from build123d import *

# Parameters (mm, degrees)
SKETCH_1_R          = 9
EXTRUDE_1_DEPTH     = 20
EXTRUDE_START       = 10
SKETCH_2_R          = 9
EXTRUDE_2_DEPTH     = 10
SKETCH_4_R          = 5.45
SKETCH_4_R_2        = 2.8
CUT_EXTRUDE_1_DEPTH = 7
SKETCH_5_R          = 2.9
EXTRUDE_3_DEPTH     = 10
CHAMFER_1_SIZE      = 0.6
CHAMFER_2_SIZE      = 0.4
FILLET_3_R          = 0.4


with BuildPart() as part:
    # 草图1 → 凸台-拉伸1 (new body)
    with BuildSketch(Plane(origin=(0, 0, 0), x_dir=(0, 0, -1), z_dir=(1, 0, 0))):
        Circle(SKETCH_1_R)
        with BuildLine():
            Line((-2.2, 4.4), (2.2, 4.4))
            Line((2.2, 4.4), (2.2, 6.8556546))
            ThreePointArc((2.2, 6.8556546), (0, -7.2), (-2.2, 6.8556546))
            Line((-2.2, 6.8556546), (-2.2, 4.4))
        make_face(mode=Mode.SUBTRACT)
    extrude(amount=-EXTRUDE_1_DEPTH)

    # 草图2 → 凸台-拉伸2 (add)
    with BuildSketch(Plane(origin=(0, 0, 0), x_dir=(0, 0, -1), z_dir=(1, 0, 0)).offset(EXTRUDE_START)):
        Circle(SKETCH_2_R)
    extrude(amount=-EXTRUDE_2_DEPTH)

    # 草图4 → 切除-拉伸1 (cut)
    with BuildSketch(Plane(origin=(10, 0, 0), x_dir=(0, 0, -1), z_dir=(1, 0, 0))):
        Circle(SKETCH_4_R)
        Circle(SKETCH_4_R_2, mode=Mode.SUBTRACT)
    extrude(amount=-CUT_EXTRUDE_1_DEPTH, mode=Mode.SUBTRACT)

    # 草图5 → 凸台-拉伸3 (add)
    with BuildSketch(Plane(origin=(10, 0, 0), x_dir=(0, 0, -1), z_dir=(1, 0, 0))):
        Circle(SKETCH_5_R)
    extrude(amount=EXTRUDE_3_DEPTH)

    # Chamfer 1
    chamfer_1_edges = [part.edges().sort_by_distance(p)[0] for p in [
        (10, 0, 5.45),
    ]]
    chamfer(chamfer_1_edges, length=CHAMFER_1_SIZE)

    # Chamfer 2
    chamfer_2_edges = [part.edges().sort_by_distance(p)[0] for p in [
        (-20, 0, 9),
        (-20, 5.6278273, 2.2),
        (-20, 4.4, 0),
        (-20, 5.6278273, -2.2),
        (-20, -7.2, 0),
    ]]
    chamfer(chamfer_2_edges, length=CHAMFER_2_SIZE)

    # 圆角3
    fillet_3_edges = [part.edges().sort_by_distance(p)[0] for p in [
        (-9.8, 4.4, 2.2),
        (-9.8, 4.4, -2.2),
    ]]
    fillet(fillet_3_edges, radius=FILLET_3_R)


solid = part.part
Here's how the part is built. I have some questions about the finished solid (model axes, mm). A direction names the side the tool comes from. Give positions to 0.01 mm unless a question says otherwise; leave off trailing zeros. Order: outer loops, then holes, each group sorted by start corner. A loop starts at its lowest first (then second) coordinate and runs counter-clockwise, first axis right, second up. Notation, with made-up numbers: M -28,37 L 27,37 A32 ccw 27,76 Z; hole C -30.5,11.25 d11. An arc over 180 degrees is marked long. Answer as a JSON object with one key per item and string values. Group by question number.
1) Please list where these lines run through material, in increasing order: L1, parallel to Y at x = -12.5, z = 0; L2, parallel to Y at x = 7.75, z = 0; L3, parallel to Z at x = -11, y = 6. Write a range as [from, to].
2) We'd pull the mould along Z, two halves only. Please class faces 4 (the flat face through (-20, 5, 0)), 5 (the cylindrical face through (6.245, 1.637, -5.198)), 6 (the cylindrical face through (-4.593, 8.923, 1.172)): pulls with the +Z half, pulls with the -Z half, needs draft (parallel to the pull), parting line crosses it, or undercut.
3) On a 3-axis mill with a long thin cutter (end or side, diameter ignored), from which of +Z, -Z, +X, -X, +Y, -Y can I reach the whole of each face in a straight line? I mean faces 1 (the flat face through (0, 0, 0)), 2 (the cylindrical face through (6.5, 0.1, 2.8)), 3 (the flat face through (10, -6, -2)). Say none if no direction works.
4) Suppose I cut it at C-C, the plane z = 0. Write out the boundary of the cut face in (x, y), plus the area to 3 significant figures.
5) Suppose I cut it at D-D, the plane x = 14. Write out the boundary of the cut face in (y, z), plus the area to 3 significant figures.
6) I'm going to push flat-ended pins straight in: pin 1 Ø3 at (x, z) = (-6.5, -3.5) entering from -Y; pin 2 Ø8 at (x, y) = (2.5, -4.5) entering from +Z; pin 3 Ø3 at (y, z) = (0.5, 0) entering from -X. Where does each tip first touch, or does it pass through?
7) Suppose I cut it at A-A, the plane y = 0. Write out the boundary of the cut face in (x, z).
8) Suppose I cut it at B-B, the plane x = -2. Write out the boundary of the cut face in (y, z).
Results found:
{
 "1": {"L1": "[-9, -7.2], [4.4, 9]", "L2": "[-9, -5.45], [-2.8, 2.8], [5.45, 9]", "L3": "[-6.71, -3.98], [-2.2, 2.2], [3.98, 6.71]"},
 "2": {"face 4": "needs draft", "face 5": "undercut", "face 6": "parting line crosses it"},
 "3": {"face 1": "-X", "face 2": "none", "face 3": "+X"},
 "4": {"outline": "M -20,-8.6 L -19.6,-9 L 10,-9 L 10,-6.05 L 9.4,-5.45 L 3,-5.45 L 3,-2.8 L 10,-2.8 L 10,-2.9 L 20,-2.9 L 20,2.9 L 10,2.9 L 10,2.8 L 3,2.8 L 3,5.45 L 9.4,5.45 L 10,6.05 L 10,9 L -19.6,9 L -20,8.6 L -20,4.8 L -19.6,4.4 L 0,4.4 L 0,-7.2 L -19.6,-7.2 L -20,-7.6 Z", "area": "328 mm²"},
 "5": {"outline": "C 0,0 d5.8", "area": "26.4 mm²"},
 "6": {"pin 1": "y = -8.77", "pin 2": "z = 8.99", "pin 3": "x = 0"},
 "7": {"outline": "M -20,-8.6 L -19.6,-9 L 10,-9 L 10,-6.05 L 9.4,-5.45 L 3,-5.45 L 3,-2.8 L 10,-2.8 L 10,-2.9 L 20,-2.9 L 20,2.9 L 10,2.9 L 10,2.8 L 3,2.8 L 3,5.45 L 9.4,5.45 L 10,6.05 L 10,9 L -19.6,9 L -20,8.6 L -20,7.6 L -19.6,7.2 L 0,7.2 L 0,-7.2 L -19.6,-7.2 L -20,-7.6 Z"},
 "8": {"outline": "C 0,0 d18; hole M 4.4,-1.8 L 4.4,1.8 A0.4 cw 4.8,2.2 L 6.86,2.2 A7.2 ccw long 6.86,-2.2 L 4.8,-2.2 A0.4 cw Z"}
}
